Here's how the part is built. I have some questions about the finished solid (model axes, mm). Face numbers are marked on the shaded views. A direction names the side the tool comes from. Round coordinates to 2 decimals unless told otherwise and drop trailing zeros. Order: outer loops, then holes, each group sorted by start corner. A loop starts at its lowest first (then second) coordinate and runs counter-clockwise, first axis right, second up. Notation, with made-up numbers: (-31.75, 63.25) - (-27.75, 63.25) arc R18 cw to (-27.75, 98.25) - close; hole circle Ø5 at (72, -7.75). An arc over 180 degrees is marked (long way). Answer as a JSON object with one key per item and string values.
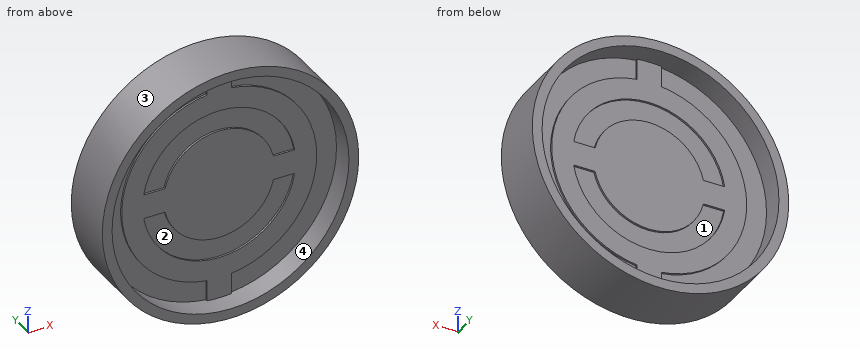
```python
from build123d import *

# Parameters (mm, degrees)
SKETCH1_R           = 15.9639
BOSS_EXTRUDE1_DEPTH = 3.4925
SKETCH2_R           = 14.7447
CUT_EXTRUDE1_DEPTH  = 2.794
BOSS_EXTRUDE2_DEPTH = 0.254


with BuildPart() as part:
    # Sketch1 → Boss-Extrude1 (new body, symmetric)
    with BuildSketch(Plane(origin=(0, 0, 0), x_dir=(1, 0, 0), z_dir=(0, 1, 0))):
        Circle(SKETCH1_R)
    extrude(amount=BOSS_EXTRUDE1_DEPTH, both=True)

    # Sketch2 → Cut-Extrude1 (cut)
    with BuildSketch(Plane(origin=(0, 3.4925, 0), x_dir=(1, 0, 0), z_dir=(0, 1, 0))):
        Circle(SKETCH2_R)
    cut_extrude1 = extrude(amount=-CUT_EXTRUDE1_DEPTH, mode=Mode.SUBTRACT)

    # Sketch3 → Boss-Extrude2 (add)
    with BuildSketch(Plane(origin=(0, 0.6985, 0), x_dir=(1, 0, 0), z_dir=(0, 1, 0))):
        with BuildLine():
            ThreePointArc((6.745125909, 1.524), (0, 6.91515), (-6.745125909, 1.524))
            Line((-6.745125909, 1.524), (-6.745125909, -1.524))
            ThreePointArc((-6.745125909, -1.524), (0, -6.91515), (6.745125909, -1.524))
            Line((6.745125909, -1.524), (6.745125909, 1.524))
        make_face()
        with BuildLine():
            ThreePointArc((-12.038771055, -1.524), (-8.580634724, -8.580634724), (-1.524, -12.038771055))
            Line((-1.524, -12.038771055), (1.524, -12.038771055))
            ThreePointArc((1.524, -12.038771055), (8.580634724, -8.580634724), (12.038771055, -1.524))
            Line((12.038771055, -1.524), (9.402289562, -1.524))
            ThreePointArc((9.402289562, -1.524), (0, -9.525), (-9.402289562, -1.524))
            Line((-9.402289562, -1.524), (-12.038771055, -1.524))
        make_face()
        with BuildLine():
            Line((1.524, 12.038771055), (-1.524, 12.038771055))
            ThreePointArc((-1.524, 12.038771055), (-8.580634724, 8.580634724), (-12.038771055, 1.524))
            Line((-12.038771055, 1.524), (-9.402289562, 1.524))
            ThreePointArc((-9.402289562, 1.524), (0, 9.525), (9.402289562, 1.524))
            Line((9.402289562, 1.524), (12.038771055, 1.524))
            ThreePointArc((12.038771055, 1.524), (8.580634724, 8.580634724), (1.524, 12.038771055))
        make_face()
        with BuildLine():
            ThreePointArc((1.524, 14.665728829), (0, 14.7447), (-1.524, 14.665728829))
            Line((-1.524, 14.665728829), (-1.524, 12.038771055))
            ThreePointArc((-1.524, 12.038771055), (0, 12.13485), (1.524, 12.038771055))
            Line((1.524, 12.038771055), (1.524, 14.665728829))
        make_face()
        with BuildLine():
            Line((-6.745125909, 1.524), (-9.402289562, 1.524))
            ThreePointArc((-9.402289562, 1.524), (-9.525, 0), (-9.402289562, -1.524))
            Line((-9.402289562, -1.524), (-6.745125909, -1.524))
            ThreePointArc((-6.745125909, -1.524), (-6.91515, 0), (-6.745125909, 1.524))
        make_face()
        with BuildLine():
            ThreePointArc((9.525, 0), (9.494272828, 0.764466129), (9.402289562, 1.524))
            Line((9.402289562, 1.524), (6.745125909, 1.524))
            ThreePointArc((6.745125909, 1.524), (6.87251253, 0.766727493), (6.91515, 0))
            ThreePointArc((6.91515, 0), (6.87251253, -0.766727493), (6.745125909, -1.524))
            Line((6.745125909, -1.524), (9.402289562, -1.524))
            ThreePointArc((9.402289562, -1.524), (9.494272828, -0.764466129), (9.525, 0))
        make_face()
        with BuildLine():
            Line((-1.524, -12.038771055), (-1.524, -14.665728829))
            ThreePointArc((-1.524, -14.665728829), (0, -14.7447), (1.524, -14.665728829))
            Line((1.524, -14.665728829), (1.524, -12.038771055))
            ThreePointArc((1.524, -12.038771055), (0, -12.13485), (-1.524, -12.038771055))
        make_face()
        with BuildLine():
            Line((-9.402289562, 1.524), (-12.038771055, 1.524))
            Line((-12.038771055, 1.524), (-12.038771055, -1.524))
            Line((-12.038771055, -1.524), (-9.402289562, -1.524))
            ThreePointArc((-9.402289562, -1.524), (-9.525, 0), (-9.402289562, 1.524))
        make_face()
        with BuildLine():
            Line((12.038771055, -1.524), (12.038771055, 1.524))
            Line((12.038771055, 1.524), (9.402289562, 1.524))
            ThreePointArc((9.402289562, 1.524), (9.494272828, 0.764466129), (9.525, 0))
            ThreePointArc((9.525, 0), (9.494272828, -0.764466129), (9.402289562, -1.524))
            Line((9.402289562, -1.524), (12.038771055, -1.524))
        make_face()
        with BuildLine():
            ThreePointArc((12.13485, 0), (12.110806444, 0.763512797), (12.038771055, 1.524))
            Line((12.038771055, 1.524), (12.038771055, -1.524))
            ThreePointArc((12.038771055, -1.524), (12.110806444, -0.763512797), (12.13485, 0))
        make_face()
        with BuildLine():
            ThreePointArc((6.91515, 0), (6.87251253, 0.766727493), (6.745125909, 1.524))
            Line((6.745125909, 1.524), (6.745125909, -1.524))
            ThreePointArc((6.745125909, -1.524), (6.87251253, -0.766727493), (6.91515, 0))
        make_face()
        with BuildLine():
            Line((-6.745125909, -1.524), (-6.745125909, 1.524))
            ThreePointArc((-6.745125909, 1.524), (-6.91515, 0), (-6.745125909, -1.524))
        make_face()
        with BuildLine():
            Line((-12.038771055, -1.524), (-12.038771055, 1.524))
            ThreePointArc((-12.038771055, 1.524), (-12.13485, 0), (-12.038771055, -1.524))
        make_face()
        with BuildLine():
            Line((1.524, -12.038771055), (-1.524, -12.038771055))
            ThreePointArc((-1.524, -12.038771055), (0, -12.13485), (1.524, -12.038771055))
        make_face()
        with BuildLine():
            ThreePointArc((1.524, 12.038771055), (0, 12.13485), (-1.524, 12.038771055))
            Line((-1.524, 12.038771055), (1.524, 12.038771055))
        make_face()
    boss_extrude2 = extrude(amount=BOSS_EXTRUDE2_DEPTH)

    # Mirror1: Cut-Extrude1, Boss-Extrude2 across plane
    add(cut_extrude1.mirror(Plane.ZX), mode=Mode.SUBTRACT)
    add(boss_extrude2.mirror(Plane.ZX))


solid = part.part
```
1. Imagine slicing it at C-C (y = 0). List the corners of the cut face in (x, z) for me, plus the area to 3 significant figures.
Responses:
{"outline": "circle Ø31.93 at (0, 0)", "area": "801 mm2"}
2. Imagine slicing it at D-D (y = 2). List the corners of the cut face in (x, z) for me.
Responses:
{"outline": "circle Ø31.93 at (0, 0); hole circle Ø29.49 at (0, 0)"}
3. For the marked faces 1 and 2, which set-ups out of +Z, -Z, +X, -X, +Y, -Y let a thin tool reach every point of the face, with its end or its side?
Responses:
{"face 1": "+Y", "face 2": "-Y"}
4. For P1, Ø4, axis at x = -6, y = -0.5, coming from the +Z side; P2, Ø1, axis at x = -7.5, z = 7, coming from the -Y side; P3, Ø12, axis at x = -9, z = -8, coming from the -Y side; P4, Ø6.5, axis at x = -6.5, z = -4.5, coming from the +Y side, each with a flat end and sliding along its axis, tell me the tip position at first contact or that it passes through.
Responses:
{"P1": "z = 15.45", "P2": "y = -0.95", "P3": "y = -3.49", "P4": "y = 0.95"}
5. If I drill on L1, parallel to X at y = -2.35, z = 0; L2, parallel to Y at x = -12, z = 8, over which ranges is the centre line in solid material (lowest first)? Write a range as [from, to].
Responses:
{"L1": "[-15.96, -14.74], [14.74, 15.96]", "L2": "[-0.7, 0.7]"}
6. Imagine slicing it at B-B (z = -13). List the corners of the cut face in (x, y) for me.
Responses:
{"outline": "(-9.27, -3.49) - (-6.96, -3.49) - (-6.96, -0.7) - (-1.52, -0.7) - (-1.52, -0.95) - (1.52, -0.95) - (1.52, -0.7) - (6.96, -0.7) - (6.96, -3.49) - (9.27, -3.49) - (9.27, 3.49) - (6.96, 3.49) - (6.96, 0.7) - (1.52, 0.7) - (1.52, 0.95) - (-1.52, 0.95) - (-1.52, 0.7) - (-6.96, 0.7) - (-6.96, 3.49) - (-9.27, 3.49) - close"}
7. Thinking about a two-plate mould opening in Z: for the marked faces 3 and 4, which applies, pulls with the +Z half, pulls with the -Z half, needs draft (parallel to the pull), parting line crosses it, or undercut?
Responses:
{"face 3": "parting line crosses it", "face 4": "undercut"}
